from build123d import *

# Parameters (mm, degrees)
F0_W     = 182.3974
F0_H     = 76.2
F1_DEPTH = 76.2
F2_W     = 38.1
F2_H     = 76.2
F3_DEPTH = 63.5
F4_R     = 38.09999
F5_R     = 12.7
F6_DEPTH = 144.2984


# Not quite as in the source:
# - a fillet or chamfer is up to 0.001 mm smaller than in the source, because OpenCascade refuses the exact size


with BuildPart() as f1:
    # F0 (on Top) → F1 (new body)
    with BuildSketch(Plane.XY):
        with Locations((91.1987, 38.1)):
            Rectangle(F0_W, F0_H)
    extrude(amount=F1_DEPTH)

    # F2 (on face) → F3 (cut)
    with BuildSketch(Plane(origin=(0, 0, 0), x_dir=(1, 0, 0), z_dir=(0, 0, -1))):
        with Locations((163.3474, -38.1)):
            Rectangle(F2_W, F2_H)
        with Locations((19.05, -38.1)):
            Rectangle(F2_W, F2_H)
    extrude(amount=-F3_DEPTH, mode=Mode.SUBTRACT)

    # F4 (radius 38.1 in the source; OpenCascade refuses exactly that, so slightly less here)
    f4_edges = [f1.edges().sort_by_distance(p)[0] for p in [
        (91.1987, 0, 0),
        (91.1987, 76.2, 0),
    ]]
    fillet(f4_edges, radius=F4_R)

    # F5 (on face) → F6 (cut, through all)
    with BuildSketch(Plane.YZ.offset(144.2974)):
        with Locations((38.1, 25.4)):
            Circle(F5_R)
    extrude(amount=-F6_DEPTH, mode=Mode.SUBTRACT)


solid = f1.part
Check sheet for the modelled part. Datum: model origin and axes. Units: mm. A direction names the side the tool comes from. Round coordinates to 2 decimals unless told otherwise and drop trailing zeros. Order: outer loops, then holes, each group sorted by start corner. A loop starts at its lowest first (then second) coordinate and runs counter-clockwise, first axis right, second up. Notation, with made-up numbers: M 48,47.5 L 85,47.5 A7 cw 85,57.5 Z; hole C 80,-22 d6. An arc over 180 degrees is marked long. One line per item, written item: value. Start each with the question number.
1. Section check D-D on y = 62. Enter the section's corners in (x, z).
2. Access from +Z, -Z, +X, -X, +Y, -Y to the whole of each face (thin tool, end or side, straight path). Record for faces 4 (the flat face through (19, 38, 63.5)), 5 (the flat face through (0, 38, 70)), 6 (the flat face through (163, 38, 63.5)).
3. Release check for a two-part mould opening along Y. For faces 1 (the cylindrical face through (91.942, 44.927, 36.109)), 2 (the cylindrical face through (91.94, 10.86, 11.46)), 3 (the flat face through (144.297, 38.6, 38.4)) record: released by +Y, released by -Y, zero draft, split by the parting line, or undercut.
4. Gauge pin test, flat ends, axial feed: P1, Ø4, axis at y = 53, z = 35, coming from the -X side; P2, Ø8, axis at x = 54.5, z = 32.5, coming from the +Y side; P3, Ø23, axis at y = 38.1, z = 25.4, coming from the -X side; P4, Ø2, axis at x = 154, y = 40.5, coming from the -Z side. Record the tip position at first contact, or that the pin passes through.
5. Scan lines: line 1 along Z through (x, y) = (73, 38); line 2 along X through (y, z) = (61, 47); line 3 along Z through (x, y) = (31, 4.5). Record each from-to range of solid material in increasing order.
6. Section check B-B on y = 34. Enter the section's corners in (x, z), and give its area (3 significant figures).
7. Section check C-C on z = 25.4. Enter the section's corners in (x, y).
Results found:
1. outline: M 0,63.5 L 38.1,63.5 L 38.1,8.43 L 144.3,8.43 L 144.3,63.5 L 182.4,63.5 L 182.4,76.2 L 0,76.2 Z
2. face 4: -Z, -X, +Y, -Y
2. face 5: +Z, -Z, -X, +Y, -Y
2. face 6: -Z, +X, +Y, -Y
3. face 1: undercut
3. face 2: released by -Y
3. face 3: zero draft
4. P1: x = 38.1
4. P2: y = 76.17
4. P3: through
4. P4: z = 63.5
5. line 1: 0 to 12.7, 38.1 to 76.2
5. line 2: 38.1 to 144.3
5. line 3: 63.5 to 76.2
6. outline: M 0,63.5 L 38.1,63.5 L 38.1,37.42 L 144.3,37.42 L 144.3,63.5 L 182.4,63.5 L 182.4,76.2 L 0,76.2 Z; M 38.1,0.22 L 144.3,0.22 L 144.3,13.38 L 38.1,13.38 Z
6. area: 6,480 mm^2
7. outline: M 38.1,2.18 L 144.3,2.18 L 144.3,25.4 L 38.1,25.4 Z; M 38.1,50.8 L 144.3,50.8 L 144.3,74.02 L 38.1,74.02 Z
